from build123d import *

# Parameters (mm, degrees)
F0_W     = 279.4
F0_H     = 279.4
F1_DEPTH = 3.175
F3_D     = 9.525


# Not quite as in the source:
# - a length typed as a fraction of an inch, garbled in the dataset ("3 / 203.2 mm" for 3/8 in), is restored


with BuildPart() as f1:
    # F0 (on Top) → F1 (new body)
    with BuildSketch(Plane.XY):
        Rectangle(F0_W, F0_H)
    extrude(amount=F1_DEPTH)

    # F3 (through all)
    with Locations(Plane.XY.offset(3.175)):
        with Locations((0, 87.9881810245), (76.2, 43.9940905122), (76.2, -43.9940905122), (0, -87.9881810245), (-76.2, -43.9940905122), (-76.2, 43.9940905122), (0, 0)):
            Hole(F3_D / 2)


solid = f1.part
Can you work these out from the model? Positions are in its coordinate system, mm. Coordinates: 2 decimals unless noted, no trailing zeros. Loops run counter-clockwise (first coordinate to the right, second up) from the corner with the lowest first, then second, coordinate; pieces in that order, holes last. Notation, with made-up numbers: (2, 17) - (46, 17) arc R23 ccw to (46, 33) - close; hole circle Ø9 at (54, -5). An arc over 180 degrees is marked (long way). Answer as a JSON object with one key per item and string values. Group by question number.
Item 1: If we section it at B-B (y = 0): List the corners of the cut face in (x, z) for me (1 decimal).
Item 2: If we section it at C-C (x = -76.2): List the corners of the cut face in (y, z) for me (3 decimals).
Item 3: If we section it at A-A (x = 0): List the corners of the cut face in (y, z) for me (1 decimal).
Item 4: If we mould it in two halves opening along X, with no side actions, what happens to faces 1 (the face through (-80.6, 42.17, 1.57)), 2 (the face through (-2, 33, 3.175))? For each: released by +X, released by -X, zero draft, split by the parting line, or undercut.
Item 5: If I drill on L1, parallel to Y at x = 0, z = 1.1; L2, parallel to X at y = -88, z = 0.6; L3, parallel to Y at x = 76.2, z = 2, over which ranges is the centre line in solid material (lowest first)? Write a range as from..to.
Item 6: For pin 1 (5.5 mm diameter, centred on x = 0, y = 0, fed in from +Z), with a flat end and sliding along its axis, tell me the tip position at first contact or that it passes through.
Returned:
{
 "1": {"outline": "(-139.7, 0) - (-4.8, 0) - (-4.8, 3.2) - (-139.7, 3.2) - close; (4.8, 0) - (139.7, 0) - (139.7, 3.2) - (4.8, 3.2) - close"},
 "2": {"outline": "(-139.7, 0) - (-48.757, 0) - (-48.757, 3.175) - (-139.7, 3.175) - close; (-39.232, 0) - (39.232, 0) - (39.232, 3.175) - (-39.232, 3.175) - close; (48.757, 0) - (139.7, 0) - (139.7, 3.175) - (48.757, 3.175) - close"},
 "3": {"outline": "(-139.7, 0) - (-92.8, 0) - (-92.8, 3.2) - (-139.7, 3.2) - close; (-83.2, 0) - (-4.8, 0) - (-4.8, 3.2) - (-83.2, 3.2) - close; (4.8, 0) - (83.2, 0) - (83.2, 3.2) - (4.8, 3.2) - close; (92.8, 0) - (139.7, 0) - (139.7, 3.2) - (92.8, 3.2) - close"},
 "4": {"face 1": "undercut", "face 2": "zero draft"},
 "5": {"L1": "y = -139.7..-92.75, -83.23..-4.76, 4.76..83.23, 92.75..139.7", "L2": "x = -139.7..-4.76, 4.76..139.7", "L3": "y = -139.7..-48.76, -39.23..39.23, 48.76..139.7"},
 "6": {"pin 1": "passes through"}
}
